Work out the finished part from the listing and answer in its coordinate system (mm). A direction names the side the tool comes from. Round coordinates to 2 decimals unless told otherwise and drop trailing zeros. Order: outer loops, then holes, each group sorted by start corner. A loop starts at its lowest first (then second) coordinate and runs counter-clockwise, first axis right, second up. Notation, with made-up numbers: (-32, 16.5) - (-27, 16.5) arc R20 ccw to (-27, 24.5) - close; hole circle Ø1 at (37.25, -22.75). An arc over 180 degrees is marked (long way). Answer in a Markdown table with one row per item.
from build123d import *

# Parameters (mm, degrees)
F3_R      = 5
F4_DEPTH  = 5
F7_DEPTH  = 11
F9_R      = 2.45
F10_DEPTH = 5
F12_R     = 0.95
F13_DEPTH = 5


# Not quite as in the source:
# - ends of sketch curves that miss each other by under 0.0002 mm in the source are joined


with BuildPart() as f1:
    # F0 (on Top) → F1 (revolve)
    with BuildSketch(Plane.XY):
        with BuildLine():
            Line((-4.5, 0), (1.5, 0))
            Line((1.5, 0), (1.5, 20))
            Line((1.5, 20), (0, 20))
            ThreePointArc((0, 20), (-1.5, 18.4999958554), (-3.0000041446, 20))
            Line((-3.0000041446, 20), (-4.5, 20))
            Line((-4.5, 20), (-4.5, 0))
        make_face()
    revolve(axis=Axis((-1.5, 0, 0), (1, 0, 0)))

    # F3 (on offset) → F4 (join)
    with BuildSketch(Plane(origin=(-4.5, 0, 0), x_dir=(0, -1, 0), z_dir=(-1, 0, 0))):
        Circle(F3_R)
    extrude(amount=F4_DEPTH)

    # F6 (on offset) → F7 (cut, through all)
    with BuildSketch(Plane(origin=(-9.5, 0, 0), x_dir=(0, -1, 0), z_dir=(-1, 0, 0))):
        with BuildLine():
            Line((1.875, 2.5), (-1.875, 2.5))
            ThreePointArc((-1.875, 2.5), (0, -3.125), (1.875, 2.5))
        make_face()
    extrude(amount=-F7_DEPTH, mode=Mode.SUBTRACT)

    # F9 (on offset) → F10 (join)
    with BuildSketch(Plane(origin=(0, 0, 2.5), x_dir=(1, 0, 0), z_dir=(0, 0, -1))):
        with Locations((-7, 0)):
            Circle(F9_R)
    extrude(amount=-F10_DEPTH)

    # F12 (on offset) → F13 (cut, through all)
    with BuildSketch(Plane.XY.offset(7.5)):
        with Locations((-7, 0)):
            Circle(F12_R)
    extrude(amount=-F13_DEPTH, mode=Mode.SUBTRACT)


solid = f1.part
1) Find section A-A, the plane y = 0. Give the vertices of the cut face in (x, z) (3 decimals), then the cut area to 3 significant figures.
Filled in:
| item | result |
|---|---|
| outline | (-9.5, -5) - (-4.5, -5) - (-4.5, -20) - (-3, -20) arc R1.5 cw to (0, -20) - (1.5, -20) - (1.5, -3.125) - (-9.5, -3.125) - close; (-9.5, 2.5) - (-7.95, 2.5) - (-7.95, 7.5) - (-9.45, 7.5) - (-9.45, 5) - (-9.5, 5) - close; (-6.05, 2.5) - (1.5, 2.5) - (1.5, 20) - (0, 20) arc R1.5 cw to (-3, 20) - (-4.5, 20) - (-4.5, 5) - (-4.55, 5) - (-4.55, 7.5) - (-6.05, 7.5) - close |
| area | 224 mm^2 |
2) The mould has two halves that part along Y. Classify faces 1 (the face through (-8.944, 1.491, 5.907)), 2 (the face through (-9.5, 0.1, -3.3)), 3 (the face through (-7.95, 0.04, 5.04)): released by +Y, released by -Y, zero draft, split by the parting line, or undercut.
Filled in:
| item | result |
|---|---|
| face 1 | split by the parting line |
| face 2 | zero draft |
| face 3 | undercut |
3) Find section D-D, the plane z = 6. Give the number of separate pieces and of enclosed holes in the cut face, then the cut area to 3 significant figures.
Filled in:
| item | result |
|---|---|
| separate pieces | 2 |
| enclosed holes | 1 |
| area | 238 mm^2 |
4) Which of the six approach directions +Z, -Z, +X, -X, +Y, -Y give full straight-line access (tool end or side, diameter ignored) to faces 4 (the face through (1.5, -4, 0)), 5 (the face through (-7, 1.1, 7.5)), 6 (the face through (-4, 0, 2.5))?
Filled in:
| item | result |
|---|---|
| face 4 | +Z, -Z, +X, +Y, -Y |
| face 5 | +Z, -X, +Y, -Y |
| face 6 | +X, -X |
5) Find section C-C, the plane x = -7. Give the vertices of the cut face in (y, z) (3 decimals), then the cut area to 3 significant figures.
Filled in:
| item | result |
|---|---|
| outline | (-2.45, 4.359) arc R5 ccw (long way) to (2.45, 4.359) - (2.45, 7.5) - (0.95, 7.5) - (0.95, 2.5) - (1.875, 2.5) arc R3.125 cw (long way) to (-1.875, 2.5) - (-0.95, 2.5) - (-0.95, 7.5) - (-2.45, 7.5) - close |
| area | 53.2 mm^2 |
6) Find section B-B, the plane z = 0. Give the vertices of the cut face in (x, y) (3 decimals), then the cut area to 3 significant figures.
Filled in:
| item | result |
|---|---|
| outline | (-9.5, -5) - (-4.5, -5) - (-4.5, -20) - (-3, -20) arc R1.5 cw to (0, -20) - (1.5, -20) - (1.5, -3.125) - (-9.5, -3.125) - close; (-9.5, 3.125) - (1.5, 3.125) - (1.5, 20) - (0, 20) arc R1.5 cw to (-3, 20) - (-4.5, 20) - (-4.5, 5) - (-9.5, 5) - close |
| area | 214 mm^2 |
7) Find the intervals of material crossed by probe 1 along Z at (x, y) = (-5.25, 0) (3 decimals); probe 2 along Y at (x, z) = (-7, 5.3); probe 3 along Z at (x, y) = (-3.25, 0) (3 decimals), in increasing order. Write a range as from..to.
Filled in:
| item | result |
|---|---|
| probe 1 | z = -5..-3.125, 2.5..7.5 |
| probe 2 | y = -2.45..-0.95, 0.95..2.45 |
| probe 3 | z = -20..-3.125, 2.5..20 |
8) Each of these flat-tipped pins is pushed along its axis until it touches: pin 1 (2 mm diameter, centred on x = -1.5, y = 0.5, fed in from -Z); pin 2 (1.5 mm diameter, centred on x = -3.5, y = 3.5, fed in from +Z); pin 3 (4 mm diameter, centred on x = -7.5, z = 5.5, fed in from +Y). Where does it stop, or does it pass through?
Filled in:
| item | result |
|---|---|
| pin 1 | stops at z = -18.88 |
| pin 2 | stops at z = 19.81 |
| pin 3 | stops at y = 3.57 |
